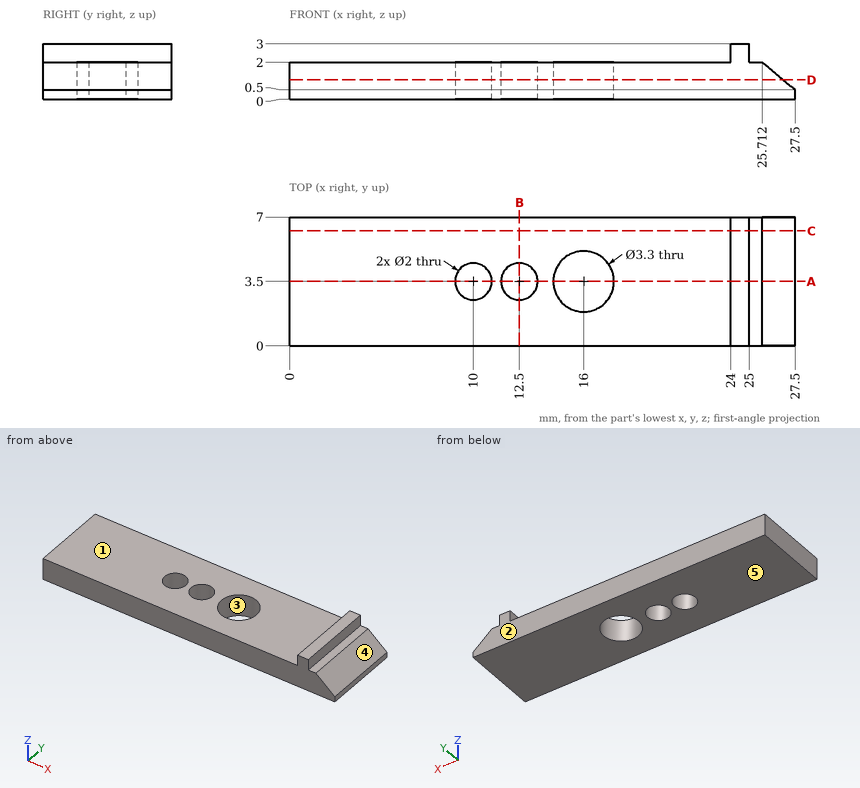
Can you work these out from the drawing? Everything is in mm from the part's minimum corner. A direction names the side the tool comes from. Round coordinates to 2 decimals unless told otherwise and drop trailing zeros. Order: outer loops, then holes, each group sorted by start corner. A loop starts at its lowest first (then second) coordinate and runs counter-clockwise, first axis right, second up.
(1) If I drill on L1, parallel to Y at x = 10, z = 1.2; L2, parallel to X at y = 3.25, z = 0.25; L3, parallel to Z at x = 19, y = 5.75, over which ranges is the centre line in solid material (lowest first)?
Results are:
L1: y = 0 to 2.5, 4.5 to 7
L2: x = 0 to 9.03, 10.97 to 11.53, 13.47 to 14.37, 17.63 to 27.5
L3: z = 0 to 2
(2) We'd pull the mould along X, two halves only. Please class the marked faces 3, 4 and 5: +X half, -X half, draft (parallel to the pull), parting line (faces both ways), or undercut.
Results are:
face 3: undercut
face 4: +X half
face 5: draft
(3) If we section it at A-A (y = 3.5): Please give me the cut outline in (x, z).
Results are:
outline: (0, 0) - (9, 0) - (9, 2) - (0, 2) - close; (11, 0) - (11.5, 0) - (11.5, 2) - (11, 2) - close; (13.5, 0) - (14.35, 0) - (14.35, 2) - (13.5, 2) - close; (17.65, 0) - (27.5, 0) - (27.5, 0.5) - (25.71, 2) - (25, 2) - (25, 3) - (24, 3) - (24, 2) - (17.65, 2) - close
(4) If we section it at C-C (y = 6.25): Please give me the cut outline in (x, z).
Results are:
outline: (0, 0) - (27.5, 0) - (27.5, 0.5) - (25.71, 2) - (25, 2) - (25, 3) - (24, 3) - (24, 2) - (0, 2) - close
(5) On a 3-axis mill with a long thin cutter (end or side, diameter ignored), from which of +Z, -Z, +X, -X, +Y, -Y can I reach the whole of each face in a straight line? I mean the marked faces 1 and 2. Say none if no direction works.
Results are:
face 1: +Z, -X, +Y, -Y
face 2: +Z, -Z, +X, -X, +Y
(6) I'm going to push flat-ended pins straight in: pin 1 (1.1 mm diameter, centred on y = 2, z = 2.5, fed in from +X); pin 2 (2 mm diameter, centred on x = 14, y = 5, fed in from +Z). Where does each tip first touch, or does it pass through?
Results are:
pin 1: stops at x = 25.77
pin 2: stops at z = 2
(7) If we section it at D-D (z = 1.05): Count the separate pieces of the cut face and the enclosed holes in it, plus the area to 3 significant figures.
Results are:
separate pieces: 1
enclosed holes: 3
area: 173 mm2
(8) If we section it at B-B (x = 12.5): Please give me the cut outline in (y, z).
Results are:
outline: (0, 0) - (2.5, 0) - (2.5, 2) - (0, 2) - close; (4.5, 0) - (7, 0) - (7, 2) - (4.5, 2) - close
